The model under review builds one solid part; all positions refer to its coordinate system, in mm. Face numbers are marked on the shaded views. A direction names the side the tool comes from. Round coordinates to 2 decimals unless told otherwise and drop trailing zeros. Order: outer loops, then holes, each group sorted by start corner. A loop starts at its lowest first (then second) coordinate and runs counter-clockwise, first axis right, second up.
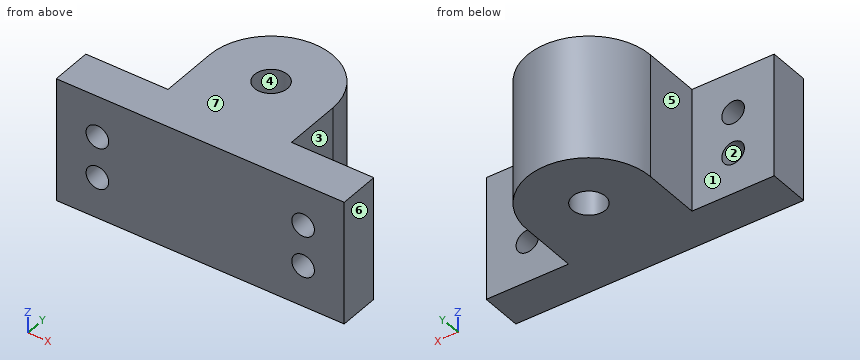
```python
from build123d import *

# Parameters (mm, degrees)
SKETCH1_R           = 2
BOSS_EXTRUDE1_DEPTH = 15
SKETCH8_W           = 15
SKETCH8_H           = 5
BOSS_EXTRUDE6_DEPTH = 10
SKETCH9_W           = 15
SKETCH9_H           = 5
BOSS_EXTRUDE7_DEPTH = 10
SKETCH10_R          = 1.375
CUT_EXTRUDE1_DEPTH  = 32.753503892


with BuildPart() as part:
    # Sketch1 → Boss-Extrude1 (new body)
    with BuildSketch(Plane.XY):
        with BuildLine():
            Line((-13.938149665, -41.724647752), (-13.938149665, -53.724647752))
            Line((-13.938149665, -53.724647752), (1.061850335, -53.724647752))
            Line((1.061850335, -53.724647752), (1.061850335, -41.724647752))
            ThreePointArc((1.061850335, -41.724647752), (-6.438149665, -34.224647752), (-13.938149665, -41.724647752))
        make_face()
        with Locations((-6.438149665, -41.724647752)):
            Circle(SKETCH1_R, mode=Mode.SUBTRACT)
    extrude(amount=BOSS_EXTRUDE1_DEPTH)

    # Sketch8 → Boss-Extrude6 (add)
    with BuildSketch(Plane.ZY.offset(13.938149665)):
        with Locations((7.5, -51.224647752)):
            Rectangle(SKETCH8_W, SKETCH8_H)
    extrude(amount=BOSS_EXTRUDE6_DEPTH)

    # Sketch9 → Boss-Extrude7 (add)
    with BuildSketch(Plane(origin=(1.061850335, 0, 0), x_dir=(0, 0, -1), z_dir=(1, 0, 0))):
        with Locations((-7.5, -51.224647752)):
            Rectangle(SKETCH9_W, SKETCH9_H)
    extrude(amount=BOSS_EXTRUDE7_DEPTH)

    # Sketch10 → Cut-Extrude1 (cut, through all)
    with BuildSketch(Plane(origin=(0, -48.724647752, 0), x_dir=(1, 0, 0), z_dir=(0, 1, 0))):
        with Locations(Location((6.061850335, -10, 0), (0, 0, 270))):
            Circle(SKETCH10_R)
        with Locations(Location((6.061850335, -5, 0), (0, 0, 270))):
            Circle(SKETCH10_R)
        with Locations(Location((-18.938149665, -10, 0), (0, 0, 270))):
            Circle(SKETCH10_R)
        with Locations(Location((-18.938149665, -5, 0), (0, 0, 270))):
            Circle(SKETCH10_R)
    extrude(amount=-CUT_EXTRUDE1_DEPTH, mode=Mode.SUBTRACT)


solid = part.part
```
(1) Draft analysis for pull direction X (two halves, no side actions). For the marked faces 4, 5, 6 and 7, state which applies: pulls with the +X half, pulls with the -X half, needs draft (parallel to the pull), parting line crosses it, or undercut.
Data:
face 4: undercut
face 5: pulls with the -X half
face 6: pulls with the +X half
face 7: needs draft
(2) Consider section B-B (z = 7). Write out the cut boundary in (x, y), and give its area (3 significant figures).
Data:
outline: (-23.94, -53.72) - (11.06, -53.72) - (11.06, -48.72) - (1.06, -48.72) - (1.06, -41.72) arc R7.5 ccw to (-13.94, -41.72) - (-13.94, -48.72) - (-23.94, -48.72) - close; hole circle Ø4 at (-6.44, -41.72)
area: 356 mm2
(3) For the marked faces 1, 2 and 3, list the 3-axis set-ups (+Z, -Z, +X, -X, +Y, -Y) from which the entire face can be reached by the end or side of a thin tool; tool diameter is ignored.
Data:
face 1: +Z, -Z, -X, +Y
face 2: +Y, -Y
face 3: +Z, -Z, +X, +Y
(4) Consider section D-D (y = -46.75). Write out the cut boundary in (x, z), and give its area (3 significant figures).
Data:
outline: (-13.94, 0) - (1.06, 0) - (1.06, 15) - (-13.94, 15) - close
area: 225 mm2
(5) To check wall thickness, follow probe 1 along X at (y, z) = (-51.85, 10); probe 2 along X at (y, z) = (-50, 3.75); probe 3 along X at (y, z) = (-46, 10.75). State the ranges of each line that lie inside material, in increasing order.
Data:
probe 1: x = -23.94 to -20.31, -17.56 to 4.69, 7.44 to 11.06
probe 2: x = -23.94 to -19.51, -18.37 to 5.49, 6.63 to 11.06
probe 3: x = -13.94 to 1.06
(6) Insertion check: pin 1 (1.6 mm diameter, centred on x = 6.06, z = 5, fed in from +Y); pin 2 (2 mm diameter, centred on y = -47, z = 9.5, fed in from +X); pin 3 (8 mm diameter, centred on x = -19.5, z = 7, fed in from +Y). Each pin has a flat end and moves straight along its axis. Give the tip position at first contact, or say it passes through.
Data:
pin 1: passes through
pin 2: stops at x = 1.06
pin 3: stops at y = -48.72
(7) Consider section C-C (y = -49.5). Write out the cut boundary in (x, z) (3 decimals), and give its area (3 significant figures).
Data:
outline: (-23.938, 0) - (11.062, 0) - (11.062, 15) - (-23.938, 15) - close; hole circle Ø2.75 at (-18.938, 5); hole circle Ø2.75 at (-18.938, 10); hole circle Ø2.75 at (6.062, 5); hole circle Ø2.75 at (6.062, 10)
area: 501 mm2
(8) Consider section A-A (z = 5). Write out the cut boundary in (x, y), and give its area (3 significant figures).
Data:
outline: (-23.94, -53.72) - (-20.31, -53.72) - (-20.31, -48.72) - (-23.94, -48.72) - close; (-17.56, -53.72) - (4.69, -53.72) - (4.69, -48.72) - (1.06, -48.72) - (1.06, -41.72) arc R7.5 ccw to (-13.94, -41.72) - (-13.94, -48.72) - (-17.56, -48.72) - close; (7.44, -53.72) - (11.06, -53.72) - (11.06, -48.72) - (7.44, -48.72) - close; hole circle Ø4 at (-6.44, -41.72)
area: 328 mm2
